Design review of the part built by this model. Coordinates are the model's own, in mm. A direction names the side the tool comes from. Give positions to 0.01 mm unless a question says otherwise; leave off trailing zeros. Order: outer loops, then holes, each group sorted by start corner. A loop starts at its lowest first (then second) coordinate and runs counter-clockwise, first axis right, second up. Notation, with made-up numbers: M 16.25,81.25 L 67.25,81.25 A21 ccw 67.25,99.25 Z; hole C 56,11 d10. An arc over 180 degrees is marked long. Put each result on its own line as item: value. Start each with the question number.
from build123d import *

# Parameters (mm, degrees)
SKETCH1_W           = 202
SKETCH1_H           = 424
BOSS_EXTRUDE1_DEPTH = 8
SKETCH2_W           = 192
SKETCH2_H           = 384
CUT_EXTRUDE1_DEPTH  = 470.727580625
SKETCH4_R           = 2
CUT_EXTRUDE2_DEPTH  = 4.78


with BuildPart() as part:
    # Sketch1 → Boss-Extrude1 (new body)
    with BuildSketch(Plane.XY):
        with Locations((101, 212)):
            Rectangle(SKETCH1_W, SKETCH1_H)
    extrude(amount=BOSS_EXTRUDE1_DEPTH)

    # Sketch2 → Cut-Extrude1 (cut, through all)
    with BuildSketch(Plane(origin=(0, 0, 0), x_dir=(-1, 0, 0), z_dir=(0, 0, -1))):
        with Locations((-101, 212)):
            Rectangle(SKETCH2_W, SKETCH2_H)
    extrude(amount=-CUT_EXTRUDE1_DEPTH, mode=Mode.SUBTRACT)

    # Sketch4 → Cut-Extrude2 (cut)
    with BuildSketch(Plane(origin=(0, 0, 0), x_dir=(-1, 0, 0), z_dir=(0, 0, -1))):
        with Locations((-184, 414)):
            Circle(SKETCH4_R)
        with Locations((-18, 414)):
            Circle(SKETCH4_R)
        with Locations((-101, 414)):
            Circle(SKETCH4_R)
    cut_extrude2 = extrude(amount=-CUT_EXTRUDE2_DEPTH, mode=Mode.SUBTRACT)

    # Mirror1: Cut-Extrude2 across plane
    add(cut_extrude2.mirror(Plane.ZX.offset(212)), mode=Mode.SUBTRACT)


solid = part.part
1. Machinability: for faces 4 (the flat face through (100, 0, 4)), 5 (the flat face through (5, 209, 4)), which of the approach directions +Z, -Z, +X, -X, +Y, -Y give a long, thin tool a straight path to every point of the face, cutting with its end or side? Answer none if there is none.
2. Consider section B-B on x = 173. Give the boundary of the cut face in (y, z), then the cut area to 3 significant figures.
3. Insertion check: pin 1 (3.5 mm diameter, centred on x = 101, y = 414, fed in from -Z); pin 2 (6.5 mm diameter, centred on x = 184, y = 414, fed in from -Z). Each pin has a flat end and moves straight along its axis. Give the tip position at first contact, or say it passes through.
4. The part is to be moulded in two halves that separate along Y. For faces 1 (the flat face through (197, 209, 4)), 2 (the flat face through (202, 209, 4)), 3 (the flat face through (100, 424, 4)), say which applies: +Y half, -Y half, draft (parallel to the pull), parting line (faces both ways), or undercut.
5. Consider section C-C on z = 2.5. Give the boundary of the cut face in (x, y), then the cut area to 3 significant figures.
6. Consider section A-A on y = 223. Give the boundary of the cut face in (x, z).
7. To check wall thickness, follow probe 1 along Y at (x, z) = (18, 2.65); probe 2 along X at (y, z) = (10, 3.55); probe 3 along X at (y, z) = (270, 3). State the ranges of each line that lie inside material, in increasing order.
Returned:
1. face 4: +Z, -Z, +X, -X, -Y
1. face 5: +Z, -Z
2. outline: M 0,0 L 20,0 L 20,8 L 0,8 Z; M 404,0 L 424,0 L 424,8 L 404,8 Z
2. area: 320 mm2
3. pin 1: stops at z = 4.78
3. pin 2: stops at z = 0
4. face 1: undercut
4. face 2: draft
4. face 3: +Y half
5. outline: M 0,0 L 202,0 L 202,424 L 0,424 Z; hole M 5,20 L 197,20 L 197,404 L 5,404 Z; hole C 18,10 d4; hole C 18,414 d4; hole C 101,10 d4; hole C 101,414 d4; hole C 184,10 d4; hole C 184,414 d4
5. area: 11,800 mm2
6. outline: M 0,0 L 5,0 L 5,8 L 0,8 Z; M 197,0 L 202,0 L 202,8 L 197,8 Z
7. probe 1: y = 0 to 8, 12 to 20, 404 to 412, 416 to 424
7. probe 2: x = 0 to 16, 20 to 99, 103 to 182, 186 to 202
7. probe 3: x = 0 to 5, 197 to 202
